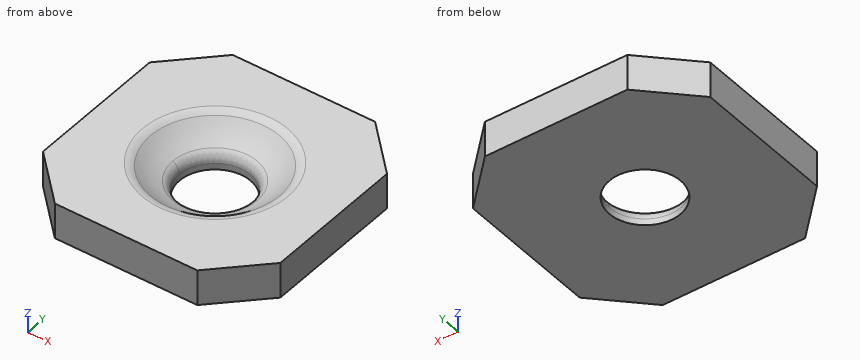
```python
from build123d import *

# Parameters (mm, degrees)
SKETCH_2_W         = 100
SKETCH_2_H         = 100
EXTRUDE_1_DEPTH    = 15
SKETCH3_R          = 15
CUT_EXTRUDE1_DEPTH = 73.284161474
CHAMFER_1_SIZE     = 20
FILLET1_R          = 5
FILLET_1_R         = 5


with BuildPart() as part:
    # ｽｹｯﾁ2 → ﾎﾞｽ - 押し出し1 (new body)
    with BuildSketch(Plane.XY):
        Rectangle(SKETCH_2_W, SKETCH_2_H)
    extrude(amount=EXTRUDE_1_DEPTH)

    # ｽｹｯﾁ3 → ｶｯﾄ - 回転1 (revolve, cut)
    with BuildSketch(Plane(origin=(0, 0, 0), x_dir=(1, 0, 0), z_dir=(0, 1, 0))):
        with BuildLine():
            Line((0, -83), (0, -3))
            ThreePointArc((0, -3), (40, -43), (0, -83))
        make_face()
    revolve(axis=Axis((0, 0, 83), (0, 0, -1)), mode=Mode.SUBTRACT)

    # Sketch3 → Cut-Extrude1 (cut, through all)
    with BuildSketch(Plane(origin=(0, 0, 0), x_dir=(-1, 0, 0), z_dir=(0, 0, -1))):
        Circle(SKETCH3_R)
    extrude(amount=-CUT_EXTRUDE1_DEPTH, mode=Mode.SUBTRACT)

    # 面取り1
    chamfer_1_edges = [part.edges().sort_by_distance(p)[0] for p in [
        (50, -50, 7.5),
        (-50, -50, 7.5),
        (-50, 50, 7.5),
        (50, 50, 7.5),
    ]]
    chamfer(chamfer_1_edges, length=CHAMFER_1_SIZE)

    # Fillet1
    fillet1_edges = [part.edges().sort_by_distance(p)[0] for p in [
        (0, -15, 5.919007565),
    ]]
    fillet(fillet1_edges, radius=FILLET1_R)

    # ﾌｨﾚｯﾄ1
    fillet_1_edges = [part.edges().sort_by_distance(p)[0] for p in [
        (-28.565713714, 0, 15),
    ]]
    fillet(fillet_1_edges, radius=FILLET_1_R)


solid = part.part
```
Read the model definition and answer for the solid it produces. Units are mm, in the model's axes. Round coordinates to 2 decimals unless told otherwise and drop trailing zeros. Write each loop counter-clockwise with the first axis right and the second up, starting at its lowest first coordinate (ties: lowest second). Pieces come first, ordered by that corner, then holes. Notation, with made-up numbers: (44.25, 32) - (73.25, 32) arc R18 ccw to (73.25, 55) - close; hole circle Ø6 at (75, 60.25). An arc over 180 degrees is marked (long way). One line per item, written item: value.
Q1. Each of these flat-tipped pins is pushed along its axis until it touches: P1, Ø1.5, axis at y = -34.5, z = 5.5, coming from the -X side; P2, Ø12, axis at x = 33, y = 20, coming from the -Z side. Where does it stop, or does it pass through?
The answers:
P1: stops at x = -46.25
P2: stops at z = 0
Q2. Straight lines are drawn through the part: line 1 (Y direction, x = 0, z = 1.3); line 2 (Z direction, x = -5.5, y = -30); line 3 (Y direction, x = -14.5, z = 6). For each, find the intervals that lie inside material, in ascending order. Write a range as from..to.
The answers:
line 1: y = -50..-15, 15..50
line 2: z = 0..15
line 3: y = -50..-7.34, 7.34..50
Q3. Find section A-A (z = 9). Determine the outline of the cut face in (x, y).
The answers:
outline: (-50, -30) - (-30, -50) - (30, -50) - (50, -30) - (50, 30) - (30, 50) - (-30, 50) - (-50, 30) - close; hole circle Ø42.14 at (0, 0)
Q4. Find section B-B (y = -40.5). Determine the outline of the cut face in (x, z).
The answers:
outline: (-39.5, 0) - (39.5, 0) - (39.5, 15) - (-39.5, 15) - close
